The listing builds one solid part. Answer for the finished solid, in the listing's coordinates (mm). A direction names the side the tool comes from. Coordinates: 2 decimals unless noted, no trailing zeros. Order: outer loops, then holes, each group sorted by start corner. A loop starts at its lowest first (then second) coordinate and runs counter-clockwise, first axis right, second up. Notation, with made-up numbers: (48, 11) - (86, 11) arc R23 cw to (86, 38) - close; hole circle Ø7 at (22, 52). An arc over 180 degrees is marked (long way). Use a Markdown table: item, result. Add a question column.
Item 1: Flat-ended cylindrical pins translate along their axes: P1, Ø1.5, axis at y = 17.5, z = 394, coming from the -X side; P2, Ø2.5, axis at y = -31.5, z = 210.5, coming from the -X side; P3, Ø5, axis at x = -85.5, z = 210.5, coming from the -Y side. Find the tip coordinate at first contact, or state that the pin passes through.
Item 2: The part is cut by section C-C, the plane y = 2. Give the vertices of the cut face in (x, z).
Item 3: The part is cut by section B-B, the plane z = 250.5. Give the vertices of the cut face in (x, y).
Item 4: The part is cut by section D-D, the plane x = 25. Give the vertices of the cut face in (y, z).
Item 5: The part is cut by section A-A, the plane x = -24.5. Give the vertices of the cut face in (y, z), then the cut area to 3 significant figures.
Item 6: Find the intervals of material crossed by line 1 along Y through (x, z) = (-35, 449); line 2 along X through (y, z) = (7.5, 191), in increasing order.
Item 7: The mould has two halves that part along Y. Classify faces 1 (the flat face through (-47, 33, 237)), 2 (the flat face through (33, 0, 237)), 3 (the flat face through (-37, -30, 237)), 4 (the flat face through (-38, -33, 237)): released by +Y, released by -Y, zero draft, split by the parting line, or undercut.
Item 8: For faces 5 (the flat face through (26.786, -19.275, 236.64)), 6 (the flat face through (24.351, 17.523, 236.64)), determine the directions among +Z, -Z, +X, -X, +Y, -Y from which every point of the face is accessible in a straight line to the end or side of a thin tool.
from build123d import *

# Parameters (mm, degrees)
BOSS_EXTRU_1_DEPTH = 480
ESQUISSE3_W        = 480
ESQUISSE3_H        = 3
BOSS_EXTRU_2_DEPTH = 20


with BuildPart() as part:
    # Esquisse1 → Boss.-Extru.1 (new body)
    with BuildSketch(Plane.XY):
        Polygon((0, 30), (-80, 30), (-80, 33), (0, 33), (5.226686531, 33), (20.395121629, 28.071476676), (33, 10.722349976), (33, -10.722349976), (20.395121629, -28.071476676), (5.226686531, -33), (0, -33), (-80, -33), (-80, -30), (0, -30), (4.75153321, -30), (18.541019662, -25.519524251), (30, -9.747590887), (30, 9.747590887), (18.541019662, 25.519524251), (4.75153321, 30), align=None)
    extrude(amount=BOSS_EXTRU_1_DEPTH)

    # Esquisse3 → Boss.-Extru.2 (add)
    with BuildSketch(Plane.ZY.offset(80)):
        with Locations((240, 31.5)):
            Rectangle(ESQUISSE3_W, ESQUISSE3_H)
    extrude(amount=BOSS_EXTRU_2_DEPTH)


solid = part.part
Solution:
| question | item | result |
|---|---|---|
| 1 | P1 | stops at x = 23.82 |
| 1 | P2 | stops at x = -80 |
| 1 | P3 | stops at y = 30 |
| 2 | outline | (30, 0) - (33, 0) - (33, 480) - (30, 480) - close |
| 3 | outline | (-100, 30) - (4.75, 30) - (18.54, 25.52) - (30, 9.75) - (30, -9.75) - (18.54, -25.52) - (4.75, -30) - (-80, -30) - (-80, -33) - (5.23, -33) - (20.4, -28.07) - (33, -10.72) - (33, 10.72) - (20.4, 28.07) - (5.23, 33) - (-100, 33) - close |
| 4 | outline | (-21.73, 0) - (-16.63, 0) - (-16.63, 480) - (-21.73, 480) - close; (16.63, 0) - (21.73, 0) - (21.73, 480) - (16.63, 480) - close |
| 5 | outline | (-33, 0) - (-30, 0) - (-30, 480) - (-33, 480) - close; (30, 0) - (33, 0) - (33, 480) - (30, 480) - close |
| 5 | area | 2,880 mm2 |
| 6 | line 1 | y = -33 to -30, 30 to 33 |
| 6 | line 2 | x = 30 to 33 |
| 7 | face 1 | released by +Y |
| 7 | face 2 | zero draft |
| 7 | face 3 | undercut |
| 7 | face 4 | released by -Y |
| 8 | face 5 | +Z, -Z, +X, -Y |
| 8 | face 6 | +Z, -Z, -X |
